from build123d import *

# Parameters (mm, degrees)
BOSS_EXTRUDE1_DEPTH = 12
SHELL1_T            = -1
SKETCH2_W           = 10
SKETCH2_H           = 10
CUT_EXTRUDE1_DEPTH  = 12
SKETCH3_R           = 2
CUT_EXTRUDE2_DEPTH  = 12
SKETCH5_W           = 0.21800788
SKETCH5_H           = 12
CUT_EXTRUDE3_DEPTH  = 1.937482958


with BuildPart() as part:
    # Sketch1 → Boss-Extrude1 (new body)
    with BuildSketch(Plane.XY):
        Polygon((-17.5, 6), (-77.342905627, -21.549973615), (-77.342905627, -35.63), (-65.906288607, -35.63), (-65.906288607, -28.284880053), (-17.5, -6), (17.5, -6), (70.263903397, -28.328632203), (70.263903397, -35.368537604), (79.19497343, -35.368537604), (79.19497343, -20.108083023), (17.5, 6), align=None)
    extrude(amount=BOSS_EXTRUDE1_DEPTH)

    # Shell1
    shell1_openings = [part.faces().sort_by_distance(p)[0] for p in [
        (-71.624597117, -35.63, 6),
    ]]
    offset(amount=SHELL1_T, openings=shell1_openings, kind=Kind.INTERSECTION)

    # Sketch2 → Cut-Extrude1 (cut)
    with BuildSketch(Plane.XZ.offset(35.63)):
        with Locations((89.157094373, 6.101364163)):
            Rectangle(SKETCH2_W, SKETCH2_H)
    extrude(amount=-CUT_EXTRUDE1_DEPTH, mode=Mode.SUBTRACT)

    # Sketch3 → Cut-Extrude2 (cut)
    with BuildSketch(Plane.XY.offset(12)):
        Circle(SKETCH3_R)
    extrude(amount=-CUT_EXTRUDE2_DEPTH, mode=Mode.SUBTRACT)

    # Sketch5 → Cut-Extrude3 (cut)
    with BuildSketch(Plane.XZ.offset(35.63)):
        with Locations((83.048090433, 6)):
            Rectangle(SKETCH5_W, SKETCH5_H)
    extrude(amount=-CUT_EXTRUDE3_DEPTH, mode=Mode.SUBTRACT)


solid = part.part
Build history of the part. All positions in model axes, mm. A direction names the side the tool comes from. Round coordinates to 2 decimals unless told otherwise and drop trailing zeros. Order: outer loops, then holes, each group sorted by start corner. A loop starts at its lowest first (then second) coordinate and runs counter-clockwise, first axis right, second up. Notation, with made-up numbers: M 18,84 L 72,84 A10 ccw 72,89 Z; hole C -32.75,-16.5 d9. An arc over 180 degrees is marked long. Use CSV: the item, a comma, the result in double quotes. Start each with the question number.
(1) Cut at D-D on y = -12. List the corners of the cut face in (x, z), then the cut area to 3 significant figures.
(2) Flat gauge pins, fed straight in: P1, Ø3, axis at x = 0, y = 0, coming from the +Z side; P2, Ø2, axis at x = 46, z = 8.5, coming from the -Y side; P3, Ø3.5, axis at x = 5.5, z = 7.5, coming from the -Y side; P4, Ø2, axis at x = 73.5, z = 8, coming from the +Y side. Where does each tip first touch, or does it go through?
(3) Drill centre lines: probe 1 along X at (y, z) = (-31, 8.75); probe 2 along Y at (x, z) = (-6, 7); probe 3 along X at (y, z) = (-20, 8). Where is each one in solid material? Low to high.
(4) Mould opens along Z. For faces 5 (the face through (-77, -35.63, 6)), 6 (the face through (71.264, -31, 6)), 7 (the face through (-42.7, -16.5, 5.9)), 8 (the face through (1, -5, 0)) say: +Z half, -Z half, draft (parallel to the pull), parting line (faces both ways), or undercut.
(5) Cut at C-C on y = 0. List the corners of the cut face in (x, z).
(6) Tool access for faces 1 (the face through (-47, -7.58, 5.92)), 2 (the face through (78.195, -28, 6)), 3 (the face through (43.513, -17.008, 5.916)), 4 (the face through (-76.343, -29, 6)): list every direction of +Z, -Z, +X, -X, +Y, -Y with a clear straight run to the whole face (end or side of a thin tool).
(7) Cut at B-B on z = 3. List the corners of the cut face in (x, y).
(8) Cut at A-A on x = 0. List the corners of the cut face in (y, z).
Findings:
1,outline,"M -56.6,0 L -30.53,0 L -30.53,12 L -56.6,12 Z; M 31.68,0 L 60.04,0 L 60.04,12 L 31.68,12 Z; hole M -54.21,1 L -32.92,1 L -32.92,11 L -54.21,11 Z; hole M 34.24,1 L 57.47,1 L 57.47,11 L 34.24,11 Z"
1,area,"208 mm^2"
2,P1,"passes through"
2,P2,"stops at y = -18.48"
2,P3,"stops at y = -6"
2,P4,"stops at y = -17.27"
3,probe 1,"x = -77.34 to -76.34, -66.91 to -65.91, 70.26 to 71.26, 78.19 to 79.19"
3,probe 2,"y = -6 to -5, 5 to 6"
3,probe 3,"x = -73.98 to -71.58, -50.3 to -47.91, 50.58 to 53.15, 76.37 to 78.94"
4,face 5,"draft"
4,face 6,"undercut"
4,face 7,"undercut"
4,face 8,"-Z half"
5,outline,"M -30.53,0 L -2,0 L -2,1 L -28.14,1 L -28.14,11 L -2,11 L -2,12 L -30.53,12 Z; M 2,0 L 31.68,0 L 31.68,12 L 2,12 L 2,11 L 29.11,11 L 29.11,1 L 2,1 Z"
6,face 1,"+Z, -Z, -X, +Y"
6,face 2,"none"
6,face 3,"+Z, -Z, -Y"
6,face 4,"-Y"
7,outline,"M -77.34,-35.63 L -76.34,-35.63 L -76.34,-22.19 L -17.28,5 L 17.3,5 L 78.19,-20.77 L 78.19,-34.37 L 71.26,-34.37 L 71.26,-27.67 L 17.7,-5 L -17.72,-5 L -66.91,-27.64 L -66.91,-35.63 L -65.91,-35.63 L -65.91,-28.28 L -17.5,-6 L 17.5,-6 L 70.26,-28.33 L 70.26,-35.37 L 79.19,-35.37 L 79.19,-20.11 L 17.5,6 L -17.5,6 L -77.34,-21.55 Z"
8,outline,"M -6,0 L -2,0 L -2,1 L -5,1 L -5,11 L -2,11 L -2,12 L -6,12 Z; M 2,0 L 6,0 L 6,12 L 2,12 L 2,11 L 5,11 L 5,1 L 2,1 Z"
